Geometry: see drawing. Coordinates: mm, zero at the bounding-box minimum. A direction names the side the tool comes from. Round coordinates to 2 decimals unless told otherwise and drop trailing zeros. Order: outer loops, then holes, each group sorted by start corner. A loop starts at its lowest first (then second) coordinate and runs counter-clockwise, first axis right, second up. Notation, with made-up numbers: (16, -10) - (38, -10) arc R21 ccw to (38, 19) - close; hole circle Ø10 at (-23, 0.25). An arc over 180 degrees is marked (long way). Put each result on its own line as item: value. Start each with the question number.
1) Access query for the marked faces 1, 2, 3 and 4. Directions: +Z, -Z, +X, -X, +Y, -Y. A direction counts if a zero-diameter tool reaches every point of the face in a straight line with its end or side. Return the directions, or none.
2) Section C-C on z = 43. Output: boundary loops of the cut face in (x, y) (1 decimal), then the cut area to 3 significant figures.
3) Section A-A on x = 86. Output: boundary loops of the cut face in (y, z) (1 decimal).
4) Line query: probe 1 along X at (y, z) = (10.5, 50) (1 decimal); probe 2 along X at (y, z) = (2, 90) (1 decimal); probe 3 along Z at (x, y) = (43.5, 7.5). Output: solid intervals per line, ascending. Write a range as [from, to].
5) Contact query for flat-ended pins moving along their axis: P1, Ø2.5, axis at y = 3.5, z = 90.5, coming from the -X side (1 decimal); P2, Ø1, axis at y = 4.5, z = 85, coming from the +X side (1 decimal); P3, Ø4, axis at x = 88, y = 2.5, coming from the +Z side (1 decimal). Output: stop coordinate, or through.
6) Mould query, pull axis Z, two halves, no side actions, for the marked faces 5, 6 and 7. Classes: +Z half, -Z half, draft (parallel to the pull), parting line (faces both ways), or undercut.
7) Section B-B on y = 3.81. State how many separate pieces and enclosed holes the cut face has, then the cut area to 3 significant figures.
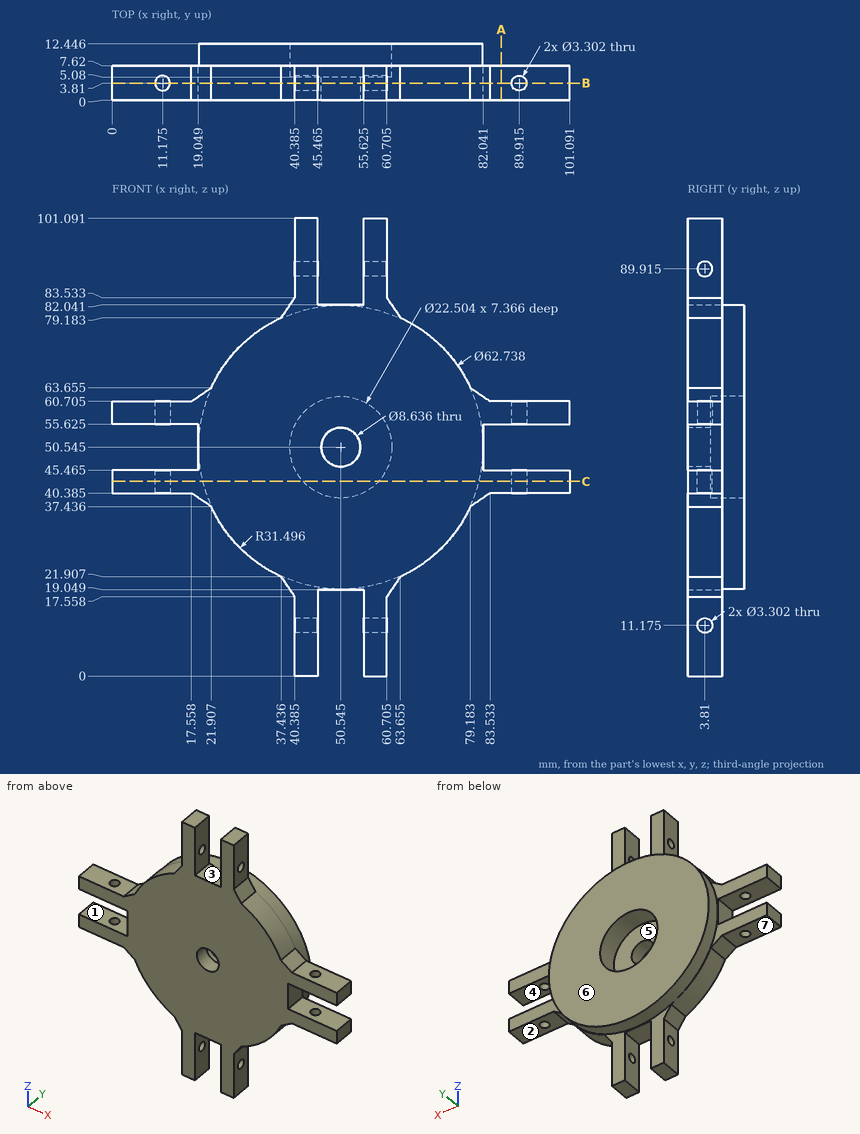
Answer sheet:
1. face 1: -X, +Y, -Y
1. face 2: -Z, +X, +Y, -Y
1. face 3: +Z, +Y, -Y
1. face 4: +X, +Y, -Y
2. outline: (0, 0) - (101.1, 0) - (101.1, 7.6) - (81, 7.6) - (81, 12.4) - (58.9, 12.4) - (58.9, 5.1) - (42.2, 5.1) - (42.2, 12.4) - (20.1, 12.4) - (20.1, 7.6) - (0, 7.6) - close; hole circle Ø3.3 at (11.2, 3.8); hole circle Ø3.3 at (89.9, 3.8)
2. area: 924 mm^2
3. outline: (0, 40.4) - (7.6, 40.4) - (7.6, 45.5) - (0, 45.5) - close; (0, 55.6) - (7.6, 55.6) - (7.6, 60.7) - (0, 60.7) - close
4. probe 1: [19.2, 39.3], [61.8, 81.9]
4. probe 2: [40.4, 45.5], [55.6, 60.7]
4. probe 3: [0, 41.77], [59.32, 101.09]
5. P1: x = 40.4
5. P2: x = 60.7
5. P3: z = 60.7
6. face 5: undercut
6. face 6: draft
6. face 7: -Z half
7. separate pieces: 9
7. enclosed holes: 1
7. area: 3,780 mm^2
